```python
from build123d import *

# Parameters (mm, degrees)
SKETCH1_R           = 3.175
SKETCH1_R_2         = 1.5875
BOSS_EXTRUDE1_DEPTH = 1.5875
FILLET1_R           = 0.127


with BuildPart() as part:
    # Sketch1 → Boss-Extrude1 (new, symmetric)
    with BuildSketch(Plane(origin=(0, 0, 0), x_dir=(1, 0, 0), z_dir=(0, 1, 0))):
        with Locations(Location((0, 0, 0), (0, 0, 270))):
            Circle(SKETCH1_R)
        with Locations(Location((0, 0, 0), (0, 0, 270))):
            Circle(SKETCH1_R_2, mode=Mode.SUBTRACT)
    extrude(amount=BOSS_EXTRUDE1_DEPTH, both=True)

    # Fillet1
    fillet1_edges = [part.edges().sort_by_distance(p)[0] for p in [
        (0, -1.5875, -3.175),
        (0, 1.5875, -3.175),
        (0, -1.5875, -1.5875),
        (0, 1.5875, -1.5875),
    ]]
    fillet(fillet1_edges, radius=FILLET1_R)


solid = part.part
```
Work out the finished part from the listing and answer in its coordinate system (mm). Give positions to 0.01 mm unless a question says otherwise; leave off trailing zeros. Use CSV: the item, a comma, the result in double quotes.
1. Flat-ended cylindrical pins translate along their axes: pin 1 Ø1.5 at (x, y) = (2, 0) entering from -Z; pin 2 Ø1.5 at (y, z) = (0, 0.5) entering from +X (3 decimals). Find the tip coordinate at first contact, or state that the pin passes through.
Found:
pin 1,"z = -2.92"
pin 2,"x = 3.175"
2. Straight lines are drawn through the part: line 1 (X direction, y = -0.1, z = 0) (1 decimal); line 2 (X direction, y = -0.4, z = 2.75); line 3 (X direction, y = 0.55, z = -1). For each, find the intervals that lie inside material, in ascending order.
Found:
line 1,"-3.2 to -1.6, 1.6 to 3.2"
line 2,"-1.59 to 1.59"
line 3,"-3.01 to -1.23, 1.23 to 3.01"
3. The mould has two halves that part along Z. Classify faces 1 (the cylindrical face through (-1.93, 0.02, -2.52)), 2 (the cylindrical face through (-0.966, -0.02, -1.26)), 3 (the flat face through (-2, 1.588, 0)): +Z half, -Z half, draft (parallel to the pull), parting line (faces both ways), or undercut.
Found:
face 1,"parting line"
face 2,"undercut"
face 3,"draft"
